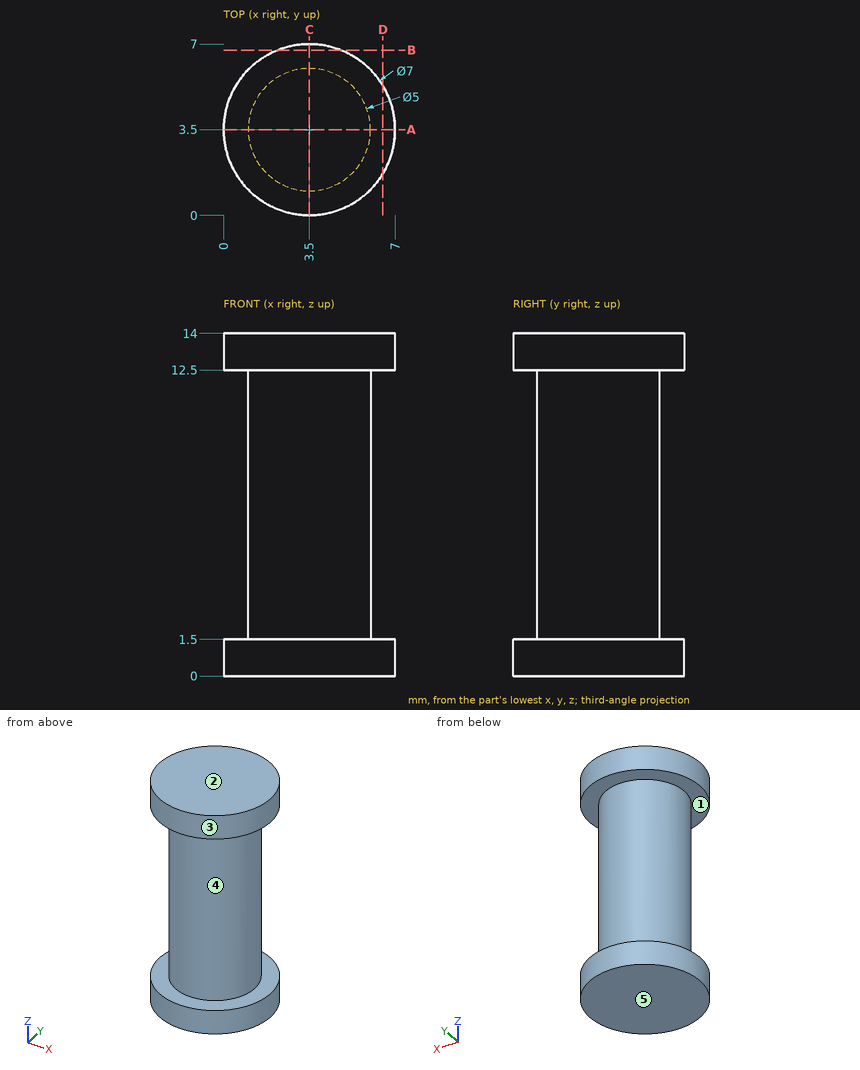
The drawing under review shows one solid part. Ordinate dimensions are in mm from its lowest x, y, z. A direction names the side the tool comes from. Round coordinates to 2 decimals unless told otherwise and drop trailing zeros. Write each loop counter-clockwise with the first axis right and the second up, starting at its lowest first coordinate (ties: lowest second). Pieces come first, ordered by that corner, then holes. Notation, with made-up numbers: (-32.5, -26) - (-8.5, -26) arc R19 cw to (-8.5, -14) - close; hole circle Ø5 at (-37, 18). An arc over 180 degrees is marked (long way). Write each question's results on one line, items separated by ' | '.
Item 1: Take a section at B-B on y = 6.75. State the section outline as (x, z) points, then the cut area to 3 significant figures.
Calculated:
outline: (2.2, 0) - (4.8, 0) - (4.8, 1.5) - (2.2, 1.5) - close; (2.2, 12.5) - (4.8, 12.5) - (4.8, 14) - (2.2, 14) - close | area: 7.79 mm^2
Item 2: Draft analysis for pull direction Z (two halves, no side actions). For the marked faces 1, 2 and 3, state which applies: pulls with the +Z half, pulls with the -Z half, needs draft (parallel to the pull), parting line crosses it, or undercut.
Calculated:
face 1: undercut | face 2: pulls with the +Z half | face 3: needs draft
Item 3: Take a section at D-D on x = 6.5. State the section outline as (y, z) points, then the cut area to 3 significant figures.
Calculated:
outline: (1.7, 0) - (5.3, 0) - (5.3, 1.5) - (1.7, 1.5) - close; (1.7, 12.5) - (5.3, 12.5) - (5.3, 14) - (1.7, 14) - close | area: 10.8 mm^2
Item 4: To check wall thickness, follow line 1 along Z through (x, y) = (6.75, 3.75); line 2 along Y through (x, z) = (3.5, 7.75); line 3 along X through (y, z) = (5.75, 4.75). State the ranges of each line that lie inside material, in increasing order. Write a range as from..to.
Calculated:
line 1: z = 0..1.5, 12.5..14 | line 2: y = 1..6 | line 3: x = 2.41..4.59
Item 5: For pin 1 (2 mm diameter, centred on x = 2, z = 8.5, fed in from -Y), flat-tipped, find the tip position at first contact; note if it passes through.
Calculated:
pin 1: stops at y = 1.05
Item 6: For the marked faces 4 and 5, list the 3-axis set-ups (+Z, -Z, +X, -X, +Y, -Y) from which the entire face can be reached by the end or side of a thin tool; tool diameter is ignored.
Calculated:
face 4: none | face 5: -Z, +X, -X, +Y, -Y
Item 7: Take a section at A-A on y = 3.5. State the section outline as (x, z) points, then the cut area to 3 significant figures.
Calculated:
outline: (0, 0) - (7, 0) - (7, 1.5) - (6, 1.5) - (6, 12.5) - (7, 12.5) - (7, 14) - (0, 14) - (0, 12.5) - (1, 12.5) - (1, 1.5) - (0, 1.5) - close | area: 76.0 mm^2
